from build123d import *

# Parameters (mm, degrees)
BOSS_EXTRU_1_DEPTH      = 10
ESQUISSE2_R             = 2.75
BOSS_EXTRU_2_DEPTH      = 3
ESQUISSE3_R             = 1.25
ENL_V_MAT_EXTRU_1_DEPTH = 8
ESQUISSE4_W             = 10
ESQUISSE4_H             = 10
BOSS_EXTRU_3_DEPTH      = 10
ENL_V_MAT_EXTRU_2_REACH = 72.178
ESQUISSE5_R             = 1.75
ESQUISSE6_R             = 3.5
ENL_V_MAT_EXTRU_3_DEPTH = 4


with BuildPart() as part:
    # Esquisse1 → Boss.-Extru.1 (new body)
    with BuildSketch(Plane.XY):
        Polygon((0, 76), (10, 76), (10, 10), (20, 10), (20, 0), (0, 0), align=None)
    extrude(amount=BOSS_EXTRU_1_DEPTH)

    # Esquisse2 → Boss.-Extru.2 (add)
    with BuildSketch(Plane.XY.offset(10)):
        with Locations(Location((5, 71, 0), (0, 0, 180))):
            Circle(ESQUISSE2_R)
        with Locations(Location((5, 5, 0), (0, 0, 180))):
            Circle(ESQUISSE2_R)
    extrude(amount=BOSS_EXTRU_2_DEPTH)

    # Esquisse3 → Enlèv. mat.-Extru.1 (cut)
    with BuildSketch(Plane.XY.offset(13)):
        with Locations((5, 71)):
            Circle(ESQUISSE3_R)
        with Locations((5, 5)):
            Circle(ESQUISSE3_R)
    extrude(amount=-ENL_V_MAT_EXTRU_1_DEPTH, mode=Mode.SUBTRACT)

    # Esquisse4 → Boss.-Extru.3 (add)
    with BuildSketch(Plane(origin=(0, 0, 0), x_dir=(-1, 0, 0), z_dir=(0, 0, -1))):
        with Locations((-5, 5)):
            Rectangle(ESQUISSE4_W, ESQUISSE4_H)
    extrude(amount=BOSS_EXTRU_3_DEPTH)

    # Esquisse5 → Enlèv. mat.-Extru.2 (cut, up to next)
    with BuildSketch(Plane(origin=(0, 10, 0), x_dir=(1, 0, 0), z_dir=(0, 1, 0)), mode=Mode.PRIVATE) as enl_v_mat_extru_2_sk1:
        with Locations(Location((15, -5, 0), (0, 0, 270))):
            Circle(ESQUISSE5_R)
    enl_v_mat_extru_2_tool1 = extrude(enl_v_mat_extru_2_sk1.sketch, amount=-ENL_V_MAT_EXTRU_2_REACH, mode=Mode.PRIVATE) & part.part
    # Esquisse5 → Enlèv. mat.-Extru.2 (cut, up to next)
    with BuildSketch(Plane(origin=(0, 10, 0), x_dir=(1, 0, 0), z_dir=(0, 1, 0)), mode=Mode.PRIVATE) as enl_v_mat_extru_2_sk2:
        with Locations(Location((5, 5, 0), (0, 0, 270))):
            Circle(ESQUISSE5_R)
    enl_v_mat_extru_2_tool2 = extrude(enl_v_mat_extru_2_sk2.sketch, amount=-ENL_V_MAT_EXTRU_2_REACH, mode=Mode.PRIVATE) & part.part
    add(enl_v_mat_extru_2_tool1.solids().sort_by_distance((15, 10, 5))[0], mode=Mode.SUBTRACT)
    add(enl_v_mat_extru_2_tool2.solids().sort_by_distance((5, 10, -5))[0], mode=Mode.SUBTRACT)

    # Esquisse6 → Enlèv. mat.-Extru.3 (cut)
    with BuildSketch(Plane(origin=(0, 10, 0), x_dir=(1, 0, 0), z_dir=(0, 1, 0))):
        with Locations(Location((15, -5, 0), (0, 0, 270))):
            Circle(ESQUISSE6_R)
        with Locations(Location((5, 5, 0), (0, 0, 270))):
            Circle(ESQUISSE6_R)
    extrude(amount=-ENL_V_MAT_EXTRU_3_DEPTH, mode=Mode.SUBTRACT)


solid = part.part
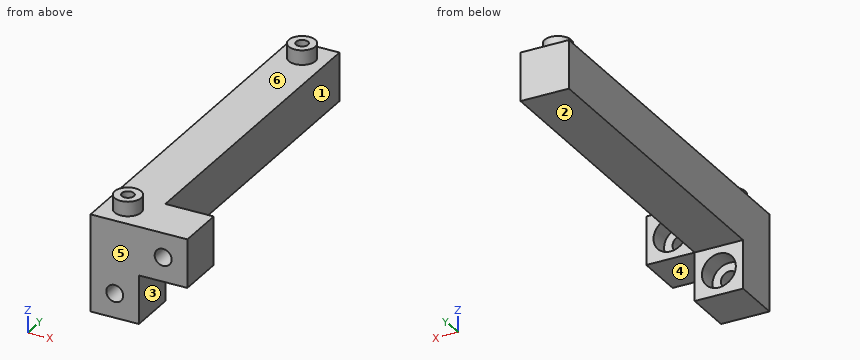
Here's how the part is built. I have some questions about the finished solid (model axes, mm). Face numbers are marked on the shaded views. A direction names the side the tool comes from. Round coordinates to 2 decimals unless told otherwise and drop trailing zeros. Write each loop counter-clockwise with the first axis right and the second up, starting at its lowest first coordinate (ties: lowest second). Pieces come first, ordered by that corner, then holes. Notation, with made-up numbers: (77.25, 44.25) -> (120.25, 44.25) arc R21 ccw to (120.25, 51.25) -> close; hole circle Ø11 at (-27.5, 20.5). An arc over 180 degrees is marked (long way). One line per item, written item: value.
1) Suppose I cut it at D-D on y = 71. List the corners of the cut face in (x, z) for me, plus the area to 3 significant figures.
Filled sheet:
outline: (0, 0) -> (10, 0) -> (10, 10) -> (7.75, 10) -> (7.75, 13) -> (6.25, 13) -> (6.25, 5) -> (3.75, 5) -> (3.75, 13) -> (2.25, 13) -> (2.25, 10) -> (0, 10) -> close
area: 96.5 mm2
2) If I drill on line 1 (Y direction, x = 5, z = 12.25); line 2 (X direction, y = 8.9, z = -5); line 3 (Y direction, x = 4.5, z = 8), over which ranges is the centre line in solid material (lowest first)? Write a range as [from, to].
Filled sheet:
line 1: y = [2.25, 3.75], [6.25, 7.75], [68.25, 69.75], [72.25, 73.75]
line 2: x = [0, 1.5], [8.5, 10]
line 3: y = [0, 3.85], [6.15, 69.85], [72.15, 76]
3) Suppose I cut it at A-A on z = -5. List the corners of the cut face in (x, y) for me.
Filled sheet:
outline: (0, 0) -> (3.25, 0) -> (3.25, 6) -> (1.5, 6) -> (1.5, 10) -> (0, 10) -> close; (6.75, 0) -> (10, 0) -> (10, 10) -> (8.5, 10) -> (8.5, 6) -> (6.75, 6) -> close
4) Suppose I cut it at C-C on z = 11. List the corners of the cut face in (x, y) for me.
Filled sheet:
outline: circle Ø5.5 at (5, 5); circle Ø5.5 at (5, 71); hole circle Ø2.5 at (5, 5); hole circle Ø2.5 at (5, 71)
5) For the marked faces 1, 2 and 3, which set-ups out of +Z, -Z, +X, -X, +Y, -Y let a thin tool reach every point of the face, with its end or its side?
Filled sheet:
face 1: +Z, -Z, +X, +Y
face 2: -Z, +X, -X, +Y
face 3: -Z, +X, +Y, -Y
6) I'm going to push flat-ended pins straight in: pin 1 Ø2 at (x, z) = (17, 0) entering from +Y; pin 2 Ø3 at (x, y) = (5, 71) entering from -Z; pin 3 Ø1.2 at (x, y) = (5, 71.5) entering from +Z. Where does each tip first touch, or does it pass through?
Filled sheet:
pin 1: stops at y = 10
pin 2: stops at z = 0
pin 3: stops at z = 5
7) We'd pull the mould along Y, two halves only. Please class the marked faces 4, 5 and 6: released by +Y, released by -Y, zero draft, split by the parting line, or undercut.
Filled sheet:
face 4: zero draft
face 5: released by -Y
face 6: undercut
8) Suppose I cut it at B-B on x = 15. List the corners of the cut face in (y, z) for me.
Filled sheet:
outline: (0, 0) -> (10, 0) -> (10, 1.5) -> (6, 1.5) -> (6, 3.25) -> (0, 3.25) -> close; (0, 6.75) -> (6, 6.75) -> (6, 8.5) -> (10, 8.5) -> (10, 10) -> (0, 10) -> close
